Here's the drawing with two shaded views (mm, measured from the low corner). I have some questions. Coordinates: 2 decimals unless noted, no trailing zeros. Order: outer loops, then holes, each group sorted by start corner. A loop starts at its lowest first (then second) coordinate and runs counter-clockwise, first axis right, second up. Notation, with made-up numbers: (-29, -24) - (-23, -24) arc R18 ccw to (-23, 7) - close; hole circle Ø4 at (20.25, 18). An arc over 180 degrees is marked (long way). Answer as a JSON object with one key per item and string values. Group by question number.
(1) Please list where these lines run through material, in increasing order: probe 1 along Y at (x, z) = (3.85, 29); probe 2 along Y at (x, z) = (3.8, 29); probe 3 along Z at (x, y) = (6.4, 39).
(2) We'd pull the mould along Z, two halves only. Please class the marked faces 1, 2 and 3: pulls with the +Z half, pulls with the -Z half, needs draft (parallel to the pull), parting line crosses it, or undercut.
(3) Imagine slicing it at D-D, the plane x = 9.5. Write out the boundary of the cut face in (y, z).
(4) Imagine slicing it at C-C, the plane x = 17.75. Write out the boundary of the cut face in (y, z), and give its area (3 significant figures).
(5) Imagine slicing it at A-A, the plane y = 29. Write out the boundary of the cut face in (x, z).
(6) Imagine slicing it at B-B, the plane x = 5.5. Write out the boundary of the cut face in (y, z), and give its area (3 significant figures).
(7) Will these pins go through, and if not, where does the flat tip stop? P1, Ø6, axis at x = 4, z = 46, coming from the -Y side; P2, Ø8, axis at x = 13.5, z = 25.5, coming from the -Y side; P3, Ø12, axis at x = 9, z = 9.5, coming from the -Y side; P4, Ø8, axis at x = 6.5, y = 38, coming from the -Z side.
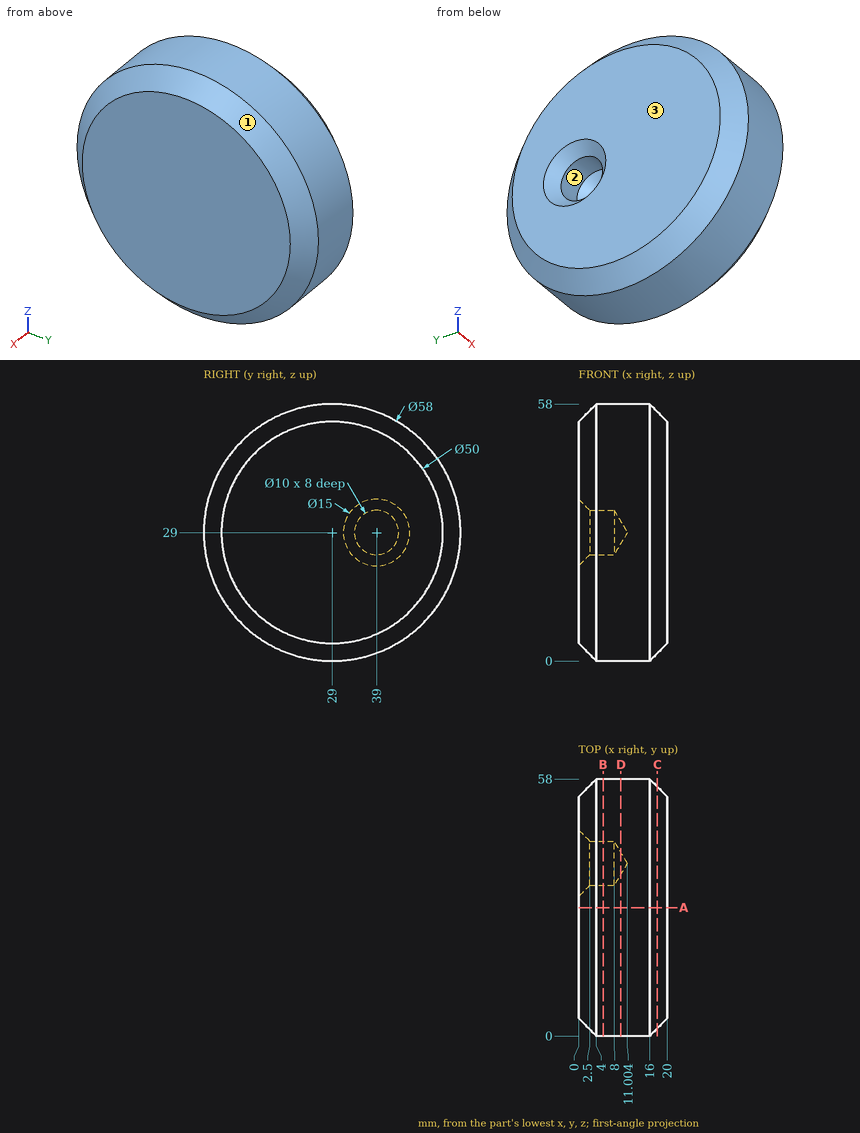
Result set:
{
 "1": {"probe 1": "y = 0.15 to 34, 44 to 57.85", "probe 2": "y = 0.2 to 34, 44 to 57.8", "probe 3": "z = 1.78 to 24, 34 to 56.22"},
 "2": {"face 1": "parting line crosses it", "face 2": "undercut", "face 3": "needs draft"},
 "3": {"outline": "circle Ø58 at (29, 29); hole circle Ø5.01 at (39, 29)"},
 "4": {"outline": "circle Ø54.5 at (29, 29)", "area": "2,330 mm^2"},
 "5": {"outline": "(0, 4) - (4, 0) - (16, 0) - (20, 4) - (20, 54) - (16, 58) - (4, 58) - (0, 54) - close"},
 "6": {"outline": "circle Ø58 at (29, 29); hole circle Ø10 at (39, 29)", "area": "2,560 mm^2"},
 "7": {"P1": "stops at y = 3.6", "P2": "stops at y = 0", "P3": "stops at y = 3.33", "P4": "stops at z = 0.43"}
}
